The listing builds one solid part. Answer for the finished solid, in the listing's coordinates (mm). A direction names the side the tool comes from. Round coordinates to 2 decimals unless told otherwise and drop trailing zeros. Write each loop counter-clockwise with the first axis right and the second up, starting at its lowest first coordinate (ties: lowest second). Pieces come first, ordered by that corner, then holes.
from build123d import *

# Parameters (mm, degrees)
F1_DEPTH  = 19.05
F2_R      = 10.16
F5_DEPTH  = 6.35
F6_DEPTH  = 69.85
F8_DEPTH  = 25.4
F10_R     = 5.08
F11_DEPTH = 0.762
F13_R     = 5.08
F14_DEPTH = 0.762
F15_R     = 0.381
F16_DEPTH = 25.4


with BuildPart() as f1:
    # F0 (on Front) → F1 (new body)
    with BuildSketch(Plane.XZ):
        with BuildLine():
            Line((31.75, 0), (31.75, 6.35))
            ThreePointArc((31.75, 6.35), (0, 8.845796), (-31.75, 6.35))
            Line((-31.75, 6.35), (-31.75, 0))
            ThreePointArc((-31.75, 0), (0, 2.495796), (31.75, 0))
        make_face()
    extrude(amount=-F1_DEPTH)

    # F2
    f2_edges = [f1.edges().sort_by_distance(p)[0] for p in [
        (-31.75, 19.05, 3.175),
        (31.75, 19.05, 3.175),
    ]]
    fillet(f2_edges, radius=F2_R)

    # F4 (on offset) → F5 (join)
    with BuildSketch(Plane.YZ.offset(31.75)):
        with BuildLine():
            Line((6.35, 1.621048), (6.35, 3.145058))
            ThreePointArc((6.35, 3.145058), (5.08, 4.415058), (3.81, 3.145058))
            Line((3.81, 3.145058), (3.81, 1.621048))
            ThreePointArc((3.81, 1.621048), (4.181974, 0.723023), (5.08, 0.351048))
            ThreePointArc((5.08, 0.351048), (5.978026, 0.723023), (6.35, 1.621048))
        make_face()
    extrude(amount=F5_DEPTH)

    # F4 (on offset) → F6 (join)
    with BuildSketch(Plane.YZ.offset(31.75)):
        with BuildLine():
            Line((6.35, 1.621048), (6.35, 3.145058))
            ThreePointArc((6.35, 3.145058), (5.08, 4.415058), (3.81, 3.145058))
            Line((3.81, 3.145058), (3.81, 1.621048))
            ThreePointArc((3.81, 1.621048), (4.181974, 0.723023), (5.08, 0.351048))
            ThreePointArc((5.08, 0.351048), (5.978026, 0.723023), (6.35, 1.621048))
        make_face()
    extrude(amount=-F6_DEPTH)

    # F7 (on Front) → F8 (cut)
    with BuildSketch(Plane.XZ):
        with BuildLine():
            Line((-31.75, 0), (31.75, 0))
            ThreePointArc((31.75, 0), (0, 2.495796), (-31.75, 0))
        make_face()
    extrude(amount=-F8_DEPTH, mode=Mode.SUBTRACT)

    # F10 (on offset) → F11 (join)
    with BuildSketch(Plane.YZ.offset(-38.1)):
        with Locations((5.08, 2.54)):
            Circle(F10_R)
    extrude(amount=F11_DEPTH)

    # F13 (on offset) → F14 (join)
    with BuildSketch(Plane.YZ.offset(38.1)):
        with Locations((5.08, 2.54)):
            Circle(F13_R)
    extrude(amount=-F14_DEPTH)

    # F15 (on Top) → F16 (cut)
    with BuildSketch(Plane.XY):
        with Locations((34.925, 5.08)):
            Circle(F15_R)
        with Locations((-34.925, 5.08)):
            Circle(F15_R)
    extrude(amount=F16_DEPTH, mode=Mode.SUBTRACT)


solid = f1.part
1. Section A-A on y = 2.5 is taken. Determine the outline of the cut face in (x, z), plus the area to 3 significant figures.
Geometry says:
outline: (-38.1, -1.84) - (-37.34, -1.84) - (-37.34, 6.92) - (-38.1, 6.92) - close; (-31.75, 0) arc R203.2 cw to (31.75, 0) - (31.75, 6.35) arc R203.2 ccw to (-31.75, 6.35) - close; (37.34, -1.84) - (38.1, -1.84) - (38.1, 6.92) - (37.34, 6.92) - close
area: 417 mm2
2. For a pull along X with two mould halves and no side action, classify faces 4 (the face through (-37.72, 9.77, 0.59)), 5 (the face through (35, 6.35, 2)), 6 (the face through (-38.1, 5, 3)) as released by +X, released by -X, zero draft, split by the parting line, or undercut.
Geometry says:
face 4: zero draft
face 5: undercut
face 6: released by -X
3. Straight lines are drawn through the part: line 1 along X through (y, z) = (5, 3.75); line 2 along X through (y, z) = (5.08, 3.55); line 3 along X through (y, z) = (3.25, -2). For each, find the intervals that lie inside material, in ascending order.
Geometry says:
line 1: x = -38.1 to -35.3, -34.55 to 34.55, 35.3 to 38.1
line 2: x = -38.1 to -35.31, -34.54 to 34.54, 35.31 to 38.1
line 3: x = -38.1 to -37.34, 37.34 to 38.1
4. A tool of negligible diameter and unlimited length cuts with its end or side. For faces 1 (the face through (35, 3.81, 2)), 2 (the face through (-34.505, 4.672, 4.348)), 3 (the face through (-35, 6.35, 2)), from which of +Z, -Z, +X, -X, +Y, -Y can it reach the whole face along a straight path? Write none if from no direction.
Geometry says:
face 1: +Z, -Z, -Y
face 2: +Z
face 3: +Z, -Z, +Y
5. Given pin 1 (6 mm diameter, centred on x = -1, y = 3, fed in from -Z); pin 2 (0.8 mm diameter, centred on x = -35.5, z = 2.5, fed in from -Y); pin 3 (8 mm diameter, centred on x = 4.5, y = 8, fed in from -Z), each flat-ended and moving along its own axis, determine where each tip first touches the part or whether it passes through.
Geometry says:
pin 1: stops at z = 2.46
pin 2: stops at y = 3.81
pin 3: stops at z = 2.32
6. Section B-B on z = -1 is taken. Determine the outline of the cut face in (x, y).
Geometry says:
outline: (-38.1, 1.44) - (-37.34, 1.44) - (-37.34, 8.72) - (-38.1, 8.72) - close; (37.34, 1.44) - (38.1, 1.44) - (38.1, 8.72) - (37.34, 8.72) - close
7. Section C-C on x = 20 is taken. Determine the outline of the cut face in (y, z), plus the area to 3 significant figures.
Geometry says:
outline: (0, 1.51) - (19.05, 1.51) - (19.05, 7.86) - (0, 7.86) - close
area: 121 mm2
8. Section D-D on x = -23 is taken. Determine the outline of the cut face in (y, z).
Geometry says:
outline: (0, 1.19) - (18.95, 1.19) - (18.95, 7.54) - (0, 7.54) - close
